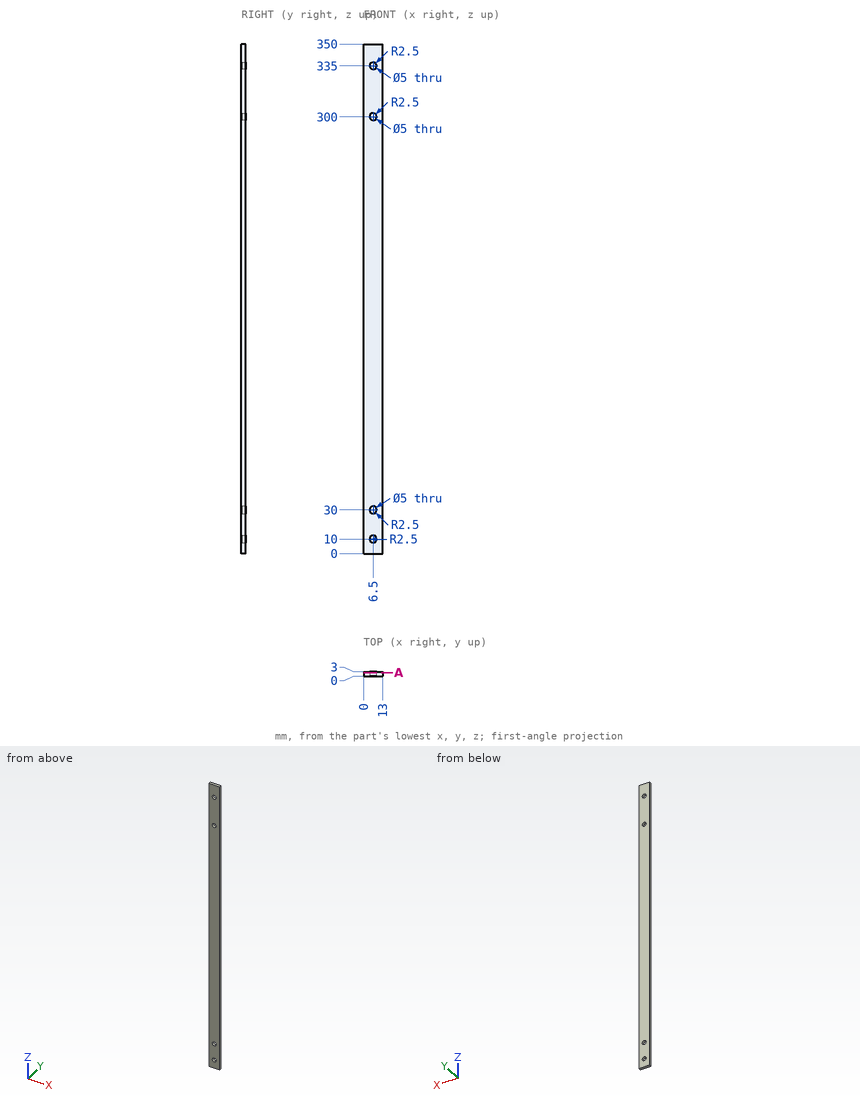
Could you check a few things on this drawing? It's one solid part, dimensions in mm from its lowest x, y, z. Round coordinates to 2 decimals unless told otherwise and drop trailing zeros. Write each loop counter-clockwise with the first axis right and the second up, starting at its lowest first coordinate (ties: lowest second). Pieces come first, ordered by that corner, then holes. Notation, with made-up numbers: (14.25, -8.75) -> (44.25, -8.75) arc R32 ccw to (44.25, 24.25) -> close; hole circle Ø1 at (57.5, -7.75). An arc over 180 degrees is marked (long way). Use one line per item in the form item = value. Start each with the question number.
Q1. I'm going to push a flat-ended pin straight in: P1, Ø4.5, axis at x = 6.5, z = 30, coming from the -Y side. Where does the tip first touch, or does it pass through?
Q2. If I drill on probe 1 along Z at (x, y) = (6.5, 2.1); probe 2 along Z at (x, y) = (8.5, 1.05); probe 3 along X at (y, z) = (2.05, 30), over which ranges is the centre line in solid material (lowest first)? Write a range as [from, to].
Q3. Imagine slicing it at A-A (y = 2.25). Please give me the cut outline in (x, z).
Worked out:
q1.P1 = through
q2.probe_1 = [0, 7.5], [12.5, 27.5], [32.5, 297.5], [302.5, 332.5], [337.5, 350]
q2.probe_2 = [0, 8.5], [11.5, 28.5], [31.5, 298.5], [301.5, 333.5], [336.5, 350]
q2.probe_3 = [0, 4], [9, 13]
q3.outline = (0, 0) -> (13, 0) -> (13, 350) -> (0, 350) -> close; hole circle Ø5 at (6.5, 10); hole circle Ø5 at (6.5, 30); hole circle Ø5 at (6.5, 300); hole circle Ø5 at (6.5, 335)
